Autodesk Fusion 360 part; units mm, degrees
sketch "Sketch2" plane through (0, 0, 0) normal (0, 0, 1) x (1, 0, 0)
  circle A0 centre (19.3, 4.7) radius 1.0002
  circle A1 centre (23.9, 4.7) radius 1
  circle A2 centre (23.9, -1.6) radius 1
  circle A3 centre (19.3, -1.6) radius 1
  circle A4 centre (11.0258, -7.3329) radius 1
  circle A5 centre (13.6665, -7.3329) radius 1
  circle A6 centre (16.2303, -7.2816) radius 1
  circle A7 centre (4.3086, -1.2823) radius 1
  circle A8 centre (4.3086, 1.3071) radius 1
  circle A9 centre (4.3086, 3.8453) radius 1
  circle A10 centre (8.2825, -4.7434) radius 1
  circle A11 centre (8.2825, 7.5628) radius 1
  circle A12 centre (18.4095, 7.5628) radius 1
  circle A13 centre (18.4095, -4.7434) radius 1
  line L0 (2, 10) -> (26, 10)
  line L1 (26, 10) -> (26, -10)
  line L2 (26, -10) -> (2, -10)
  line L3 (2, -10) -> (2, 10)
  dimension "d1" = 2
  dimension "d2" = 2
  dimension "d3" = 2
  dimension "d4" = 2
  dimension "d5" = 2
  dimension "d6" = 2
  dimension "d7" = 2
  dimension "d8" = 2
  dimension "d9" = 2
  dimension "d10" = 2
  dimension "d11" = 2
  dimension "d12" = 2
extrude "Extrude1" add sketch "Sketch2" along normal blind 1
sketch "Sketch3" plane through (0, 0, 0) normal (0, 0, 1) x (1, 0, 0)
  line L0 (8.3, -8.5) -> (18.3, -8.5)
  line L1 (18.3, -8.5) -> (18.3, -4.6)
  line L2 (18.3, -4.6) -> (8.3, -4.6)
  line L3 (8.3, -4.6) -> (8.3, -8.5)
  line L4 (3.1366, 6.2847) -> (6.7858, 6.2847)
  line L5 (6.7858, 6.2847) -> (6.7858, -3.5343)
  line L6 (6.7858, -3.5343) -> (3.1366, -3.5343)
  line L7 (3.1366, -3.5343) -> (3.1366, 6.2847)
  line L8 (6.5, -5) -> (20, -5)
  line L9 (20, -5) -> (20, 9)
  line L10 (20, 9) -> (6.5, 9)
  line L11 (6.5, 9) -> (6.5, -5)
  line L12 (20, -3) -> (25.5, -3)
  line L13 (25.5, -3) -> (25.5, 6.5)
  line L14 (25.5, 6.5) -> (20, 6.5)
  line L15 (20, 6.5) -> (20, -3)
  line L16 (10.2456, 9) -> (16.0175, 9)
  line L17 (16.0175, 9) -> (16.0175, 8.206)
  line L18 (16.0175, 8.206) -> (10.2456, 8.206)
  line L19 (10.2456, 8.206) -> (10.2456, 9)
  line L20 (2, -10) -> (26, -10)
  line L21 (26, -10) -> (26, 10)
  line L22 (26, 10) -> (2, 10)
  line L23 (2, 10) -> (2, -10)
  line L24 (20, -5) -> (6.5, -5)
  line L25 (6.5, -5) -> (6.5, -6)
  line L26 (6.5, -6) -> (20, -6)
  line L27 (20, -6) -> (20, -5)
extrude "Extrude2" add sketch "Sketch3" against normal blind 1 contours L10 L16 L17 L18 L19 | L20 L21 L22 L23
sketch "Sketch4" plane through (0, 0, 0) normal (0, 0, 1) x (1, 0, 0)
  circle A0 centre (13.3, 1.5) radius 0.7133
  line L0 (13.3, 1.5) -> (28.3, 1.5)
  line L1 (28.3, 1.5) -> (28.3, 14)
  line L2 (28.3, 14) -> (13.3, 14)
  line L3 (13.3, 14) -> (13.3, 1.5)
  line L4 (13.3, 1.5) -> (28.3, 1.5)
  line L5 (28.3, 1.5) -> (28.3, -11)
  line L6 (28.3, -11) -> (13.3, -11)
  line L7 (13.3, -11) -> (13.3, 1.5)
  line L8 (13.3, 1.5) -> (-1.7, 1.5)
  line L9 (-1.7, 1.5) -> (-1.7, 14)
  line L10 (-1.7, 14) -> (13.3, 14)
  line L11 (13.3, 14) -> (13.3, 1.5)
  line L12 (13.3, 1.5) -> (-1.7, 1.5)
  line L13 (-1.7, 1.5) -> (-1.7, -11)
  line L14 (-1.7, -11) -> (13.3, -11)
  line L15 (13.3, -11) -> (13.3, 1.5)
  line L16 (26, 10) -> (2, 10)
  line L17 (2, 10) -> (2, -10)
  line L18 (2, -10) -> (26, -10)
  line L19 (26, -10) -> (26, 10)
  dimension "d19" = 15
  dimension "d20" = 12.5
  dimension "d21" = 15
  dimension "d22" = 12.5
  dimension "d23" = 15
  dimension "d24" = 12.5
  dimension "d25" = 15
  dimension "d26" = 12.5
extrude "Extrude3" add sketch "Sketch4" along normal blind 1 contours L0 L1 L2 L3 L4 L11 L16 L19 | L0 L4 L5 L6 L7 L15 L18 L19 | L3 L8 L9 L10 L11 L12 L16 L17 | L7 L8 L12 L13 L14 L15 L17 L18
extrude "Extrude4" add 1 faces at (9.5333, 12.6667, 0) along direction (0, 0, -1) blind 1
sketch "Sketch5" plane through (0, 0, -1) normal (0, 0, -1) x (1, 0, 0)
  line L0 (-1.7, 11) -> (-1.7, -14)
  line L1 (-1.7, -14) -> (28.3, -14)
  line L2 (28.3, -14) -> (28.3, 11)
  line L3 (28.3, 11) -> (-1.7, 11)
  line L4 (6.5, 3.5343) -> (6.5, 6)
  line L5 (6.5, 6) -> (8.3, 6)
  line L6 (8.3, 6) -> (8.3, 8.5)
  line L7 (8.3, 8.5) -> (18.3, 8.5)
  line L8 (18.3, 8.5) -> (18.3, 6)
  line L9 (18.3, 6) -> (20, 6)
  line L10 (20, 6) -> (20, 3)
  line L11 (20, 3) -> (25.5, 3)
  line L12 (25.5, 3) -> (25.5, -6.5)
  line L13 (25.5, -6.5) -> (20, -6.5)
  line L14 (20, -6.5) -> (20, -9)
  line L15 (20, -9) -> (16.0175, -9)
  line L16 (16.0175, -9) -> (16.0175, -8.206)
  line L17 (16.0175, -8.206) -> (10.2456, -8.206)
  line L18 (10.2456, -8.206) -> (10.2456, -9)
  line L19 (10.2456, -9) -> (6.5, -9)
  line L20 (6.5, -9) -> (6.5, -6.2847)
  line L21 (6.5, -6.2847) -> (3.1366, -6.2847)
  line L22 (3.1366, -6.2847) -> (3.1366, 3.5343)
  line L23 (3.1366, 3.5343) -> (6.5, 3.5343)
  line L24 (28.3, -14) -> (22.3, -14)
  line L25 (22.3, -14) -> (22.3, -8)
  line L26 (22.3, -8) -> (28.3, -8)
  line L27 (28.3, -8) -> (28.3, -14)
  circle A0 centre (22.3, -8) radius 1
  line L28 (28.3, 11) -> (22.3, 11)
  line L29 (22.3, 11) -> (22.3, 5)
  line L30 (22.3, 5) -> (28.3, 5)
  line L31 (28.3, 5) -> (28.3, 11)
  circle A1 centre (22.3, 5) radius 1
  line L32 (-1.7, -14) -> (4.3, -14)
  line L33 (4.3, -14) -> (4.3, -8)
  line L34 (4.3, -8) -> (-1.7, -8)
  line L35 (-1.7, -8) -> (-1.7, -14)
  circle A2 centre (4.3, -8) radius 1
  line L36 (-1.7, 11) -> (4.3, 11)
  line L37 (4.3, 11) -> (4.3, 5)
  line L38 (4.3, 5) -> (-1.7, 5)
  line L39 (-1.7, 5) -> (-1.7, 11)
  circle A3 centre (4.3, 5) radius 1
  dimension "d31" = 2
  dimension "d32" = 2
  dimension "d33" = 6
  dimension "d34" = 6
  dimension "d35" = 2
  dimension "d36" = 6
  dimension "d37" = 2
  dimension "d40" = 6
  dimension "d43" = 6
  dimension "d44" = 6
  dimension "d45" = 6
  dimension "d46" = 6
extrude "Extrude5" cut sketch "Sketch5" against normal blind 2 contours L37 L38 A3 | L37 L38 A3 | L33 L34 A2 | L33 L34 A2 | L29 L30 A1 | L29 L30 A1 | L25 L26 A0 | L25 L26 A0
sketch "Sketch6" plane through (0, 0, -1) normal (0, 0, -1) x (1, 0, 0)
  circle A0 centre (4.3, 5) radius 1
  circle A1 centre (22.3, -8) radius 1
  circle A2 centre (4.3, -8) radius 1
  circle A3 centre (22.3, 5) radius 1
  line L0 (-1.7, 11) -> (-1.7, -14)
  line L1 (-1.7, -14) -> (28.3, -14)
  line L2 (28.3, -14) -> (28.3, 11)
  line L3 (28.3, 11) -> (-1.7, 11)
  line L4 (6.5, 3.5343) -> (6.5, 6)
  line L5 (6.5, 6) -> (8.3, 6)
  line L6 (8.3, 6) -> (8.3, 8.5)
  line L7 (8.3, 8.5) -> (18.3, 8.5)
  line L8 (18.3, 8.5) -> (18.3, 6)
  line L9 (18.3, 6) -> (20, 6)
  line L10 (20, 6) -> (20, 3)
  line L11 (20, 3) -> (25.5, 3)
  line L12 (25.5, 3) -> (25.5, -6.5)
  line L13 (25.5, -6.5) -> (20, -6.5)
  line L14 (20, -6.5) -> (20, -9)
  line L15 (20, -9) -> (16.0175, -9)
  line L16 (16.0175, -9) -> (16.0175, -8.206)
  line L17 (16.0175, -8.206) -> (10.2456, -8.206)
  line L18 (10.2456, -8.206) -> (10.2456, -9)
  line L19 (10.2456, -9) -> (6.5, -9)
  line L20 (6.5, -9) -> (6.5, -6.2847)
  line L21 (6.5, -6.2847) -> (3.1366, -6.2847)
  line L22 (3.1366, -6.2847) -> (3.1366, 3.5343)
  line L23 (3.1366, 3.5343) -> (6.5, 3.5343)
  circle A4 centre (13.3696, -1.5612) radius 15.0697
extrude "Extrude6" cut sketch "Sketch6" against normal blind 2 contours L0 L3 A4 | L0 L1 A4 | L2 L3 A4 | L1 L2 A4
equation "d33 = distanceFromRightLeft"
equation "d34 = distanceFromRightLeft"
equation "d36 = distanceFromRightLeft"
equation "d40 = distanceFromTopDown"
equation "distanceFromRightLeft = 6 mm"
equation "distanceFromTopDown = 6 mm"
equation "d43 = distanceFromTopDown"
equation "d44 = distanceFromRightLeft"
equation "d45 = distanceFromTopDown"
equation "d46 = distanceFromTopDown"
Could you check a few things on this model? Use its own coordinates, in mm. A direction names the side the tool comes from. Round coordinates to 2 decimals unless told otherwise and drop trailing zeros. Write each loop counter-clockwise with the first axis right and the second up, starting at its lowest first coordinate (ties: lowest second). Pieces come first, ordered by that corner, then holes. Notation, with made-up numbers: (22.5, 50.25) - (57.5, 50.25) arc R9 cw to (57.5, 55.25) - close; hole circle Ø8 at (15, -10). An arc over 180 degrees is marked (long way). Put each result on its own line as item: value. Start each with the question number.
(1) I want a section at A-A, the plane x = 23.9. Please give me the cut outline in (y, z).
(2) For faces 4 (the flat face through (6, 7, -1)), 5 (the flat face through (18.3, -7.3, -0.5)), which set-ups out of +Z, -Z, +X, -X, +Y, -Y let a thin tool reach every point of the face, with its end or its side?
(3) I want a section at B-B, the plane x = 4. Please give me the cut outline in (y, z).
(4) I want a section at C-C, the plane z = 0.4. Give the number of separate pieces and of enclosed holes in the cut face, plus the area to 3 significant figures.
(5) Will these pins go through, and if not, where does the flat tip stop? pin 1 (1 mm diameter, centred on y = -2, z = 0, fed in from -X); pin 2 (0.5 mm diameter, centred on y = 8, z = -0.5, fed in from -X).
(6) I need wall thicknesses on probe 1 along Y at (x, z) = (18, -0.15); probe 2 along X at (y, z) = (8.5, -0.3); probe 3 along Y at (x, z) = (22, 0.9). Which ranges of each line are inside material? Lowest first, please.
(7) Thinking about a two-plate mould opening in X: for faces 1 (the cylindrical face through (26.14, 9.56, -0.01)), 2 (the flat face through (13, 2, 1)), 3 (the cylindrical face through (3.31, 1.26, 0.49)), which applies, released by +X, released by -X, zero draft, split by the parting line, or undercut?
Here are the results:
1. outline: (-9.22, -1) - (-3, -1) - (-3, 0) - (-2.6, 0) - (-2.6, 1) - (-9.22, 1) - close; (-0.6, 0) - (3.7, 0) - (3.7, 1) - (-0.6, 1) - close; (5.7, 0) - (6.5, 0) - (6.5, -1) - (12.34, -1) - (12.34, 1) - (5.7, 1) - close
2. face 4: -Z, +X, -X, +Y, -Y
2. face 5: -Z
3. outline: (-10.24, -1) - (-5.95, -1) - (-5.95, 1) - (-10.24, 1) - close; (-4.05, -1) - (-3.53, -1) - (-3.53, 0) - (-2.23, 0) - (-2.23, 1) - (-4.05, 1) - close; (-0.33, 0) - (0.36, 0) - (0.36, 1) - (-0.33, 1) - close; (2.26, 0) - (2.89, 0) - (2.89, 1) - (2.26, 1) - close; (4.8, 0) - (6.28, 0) - (6.28, -1) - (7.05, -1) - (7.05, 1) - (4.8, 1) - close; (8.95, -1) - (13.36, -1) - (13.36, 1) - (8.95, 1) - close
4. separate pieces: 1
4. enclosed holes: 18
4. area: 598 mm^2
5. pin 1: stops at x = -1.39
5. pin 2: stops at x = -0.37
6. probe 1: y = -11 to -8.5, 9 to 14
6. probe 2: x = -0.01 to 3.43, 5.17 to 6.5, 10.25 to 16.02, 20 to 21.43, 23.17 to 26.75
6. probe 3: y = -10.79 to -5.95, -4.05 to 7.05, 8.95 to 13.91
7. face 1: released by +X
7. face 2: zero draft
7. face 3: undercut
